from build123d import *

# Parameters (mm, degrees)
SKETCH1_W           = 5.35
SKETCH1_H           = 8.5
BOSS_EXTRUDE1_DEPTH = 12.35
SKETCH2_W           = 2.75
SKETCH2_H           = 2.75
BOSS_EXTRUDE2_DEPTH = 10
SKETCH4_W           = 4.7
SKETCH4_H           = 4.65
BOSS_EXTRUDE4_DEPTH = 6
SKETCH3_R           = 0.5
BOSS_EXTRUDE3_DEPTH = 3.2


with BuildPart() as part:
    # Sketch1 → Boss-Extrude1 (new body)
    with BuildSketch(Plane.XY):
        Rectangle(SKETCH1_W, SKETCH1_H)
    extrude(amount=BOSS_EXTRUDE1_DEPTH)

    # Sketch2 → Boss-Extrude2 (add)
    with BuildSketch(Plane.XY.offset(12.35)):
        Rectangle(SKETCH2_W, SKETCH2_H)
    extrude(amount=BOSS_EXTRUDE2_DEPTH)

    # Sketch4 → Boss-Extrude4 (add)
    with BuildSketch(Plane.XY.offset(12.35)):
        with Locations((0, -0.075)):
            Rectangle(SKETCH4_W, SKETCH4_H)
    extrude(amount=BOSS_EXTRUDE4_DEPTH)

    # Sketch3 → Boss-Extrude3 (add)
    with BuildSketch(Plane.XZ.offset(4.25)):
        with Locations(Location((0, 8.6, 0), (0, 0, 90))):
            Circle(SKETCH3_R)
        with Locations(Location((0, 6.06, 0), (0, 0, 90))):
            Circle(SKETCH3_R)
        with Locations(Location((0, 3.52, 0), (0, 0, 90))):
            Circle(SKETCH3_R)
    extrude(amount=BOSS_EXTRUDE3_DEPTH)


solid = part.part
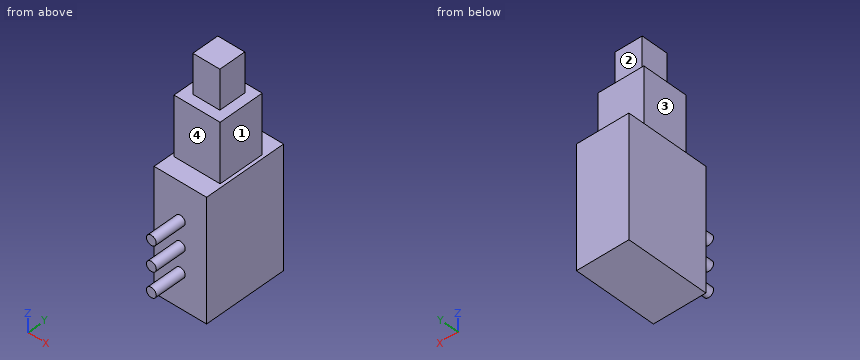
Design review of the part built by this model. Coordinates are the model's own, in mm. Face numbers are marked on the shaded views. A direction names the side the tool comes from. Give positions to 0.01 mm unless a question says otherwise; leave off trailing zeros. Order: outer loops, then holes, each group sorted by start corner. A loop starts at its lowest first (then second) coordinate and runs counter-clockwise, first axis right, second up.
1. To check wall thickness, follow L1, parallel to Z at x = 2.15, y = 0.75; L2, parallel to Y at x = -1.45, z = 1.5; L3, parallel to X at y = -1.5, z = 12.5. State the ranges of each line that lie inside material, in increasing order.
Solution:
L1: z = 0 to 18.35
L2: y = -4.25 to 4.25
L3: x = -2.35 to 2.35
2. Tool access review of the marked faces 1, 2, 3 and 4: name each direction out of +Z, -Z, +X, -X, +Y, -Y from which nothing blocks a thin tool from reaching the whole face with its end or side.
Solution:
face 1: +Z, +X, +Y, -Y
face 2: +Z, +X, -X, +Y
face 3: +Z, -X, +Y, -Y
face 4: +Z, +X, -X, -Y
3. Add section B-B, the plane x = 0. State the section outline as (y, z) points (3 decimals), then the cut area to 3 significant figures.
Solution:
outline: (-7.45, 3.02) - (-4.25, 3.02) - (-4.25, 0) - (4.25, 0) - (4.25, 12.35) - (2.25, 12.35) - (2.25, 18.35) - (1.375, 18.35) - (1.375, 22.35) - (-1.375, 22.35) - (-1.375, 18.35) - (-2.4, 18.35) - (-2.4, 12.35) - (-4.25, 12.35) - (-4.25, 9.1) - (-7.45, 9.1) - (-7.45, 8.1) - (-4.25, 8.1) - (-4.25, 6.56) - (-7.45, 6.56) - (-7.45, 5.56) - (-4.25, 5.56) - (-4.25, 4.02) - (-7.45, 4.02) - close
area: 153 mm2
4. For pin 1 Ø5 at (y, z) = (0.5, 15.5) entering from -X; pin 2 Ø3 at (x, z) = (-1.5, 15) entering from -Y; pin 3 Ø0.8 at (x, z) = (0, 20.5) entering from +Y (3 decimals), all flat-tipped, find the tip position at first contact; note any pin that passes through.
Solution:
pin 1: stops at x = -2.35
pin 2: stops at y = -2.4
pin 3: stops at y = 1.375
5. Add section A-A, the plane z = 6.06. State the section outline as (x, y) points (3 decimals), then the cut area to 3 significant figures.
Solution:
outline: (-2.675, -4.25) - (-0.5, -4.25) - (-0.5, -7.45) - (0.5, -7.45) - (0.5, -4.25) - (2.675, -4.25) - (2.675, 4.25) - (-2.675, 4.25) - close
area: 48.7 mm2
6. Add section C-C, the plane y = -0.25. State the section outline as (x, z) points (3 decimals).
Solution:
outline: (-2.675, 0) - (2.675, 0) - (2.675, 12.35) - (2.35, 12.35) - (2.35, 18.35) - (1.375, 18.35) - (1.375, 22.35) - (-1.375, 22.35) - (-1.375, 18.35) - (-2.35, 18.35) - (-2.35, 12.35) - (-2.675, 12.35) - close
7. Add section D-D, the plane y = -4.5. State the section outline as (x, z) points.
Solution:
outline: circle Ø1 at (0, 3.52); circle Ø1 at (0, 6.06); circle Ø1 at (0, 8.6)
